from build123d import *

# Parameters (mm, degrees)
SKETCH1_R           = 27.5
SKETCH1_R_2         = 15.5
BOSS_EXTRUDE1_DEPTH = 9
BOSS_EXTRUDE2_DEPTH = 9
SKETCH3_W           = 14
SKETCH3_H           = 2
SKETCH4_W           = 1.6
SKETCH4_H           = 1.9
FILLET1_R           = 10
SKETCH5_W           = 16
SKETCH5_H           = 1
CUT_EXTRUDE1_DEPTH  = 60
SKETCH6_R           = 3
CUT_EXTRUDE2_DEPTH  = 107.495305061
SKETCH7_R           = 3
CUT_EXTRUDE3_DEPTH  = 107.495305061


with BuildPart() as part:
    # Sketch1 → Boss-Extrude1 (new, symmetric)
    with BuildSketch(Plane.XY):
        Circle(SKETCH1_R)
        Circle(SKETCH1_R_2, mode=Mode.SUBTRACT)
    extrude(amount=BOSS_EXTRUDE1_DEPTH, both=True)

    # Sketch2 → Boss-Extrude2 (add, symmetric)
    with BuildSketch(Plane.XY):
        Polygon((-8, 100), (8, 100), (8, 26.310644234), (0, 27.5), (-8, 26.310644234), align=None)
    boss_extrude2 = extrude(amount=BOSS_EXTRUDE2_DEPTH, both=True)

    # Mirror1: Boss-Extrude2 across plane
    add(boss_extrude2.mirror(Plane.ZX))

    # Sketch3 → Cut-Revolve1 (revolve, cut)
    with BuildSketch(Plane(origin=(0, 0, 0), x_dir=(0, 0, -1), z_dir=(1, 0, 0)), mode=Mode.PRIVATE) as cut_revolve1_sk:
        with Locations((-2, 16.5)):
            Rectangle(SKETCH3_W, SKETCH3_H)
    revolve(cut_revolve1_sk.sketch.rotate(Axis((0, 0, 0), (0, 0, -1)), 90), axis=Axis((0, 0, 0), (0, 0, -1)), mode=Mode.SUBTRACT)

    # Sketch4 → Cut-Revolve2 (revolve, cut)
    with BuildSketch(Plane(origin=(0, 0, 0), x_dir=(0, 0, -1), z_dir=(1, 0, 0)), mode=Mode.PRIVATE) as cut_revolve2_sk:
        with Locations((-5.7, 17.95)):
            Rectangle(SKETCH4_W, SKETCH4_H)
    revolve(cut_revolve2_sk.sketch.rotate(Axis((0, 0, 0), (0, 0, -1)), 90), axis=Axis((0, 0, 0), (0, 0, -1)), mode=Mode.SUBTRACT)

    # Fillet1
    fillet1_edges = [part.edges().sort_by_distance(p)[0] for p in [
        (8, 26.310644234, 0),
        (-8, 26.310644234, 0),
        (8, -26.310644234, 0),
        (-8, -26.310644234, 0),
    ]]
    fillet(fillet1_edges, radius=FILLET1_R)

    # Sketch5 → Cut-Extrude1 (cut)
    with BuildSketch(Plane.XZ.offset(100)):
        with Locations((0, 8.5)):
            Rectangle(SKETCH5_W, SKETCH5_H)
        with Locations((0, -8.5)):
            Rectangle(SKETCH5_W, SKETCH5_H)
    cut_extrude1 = extrude(amount=-CUT_EXTRUDE1_DEPTH, mode=Mode.SUBTRACT)

    # Sketch6 → Cut-Extrude2 (cut, through all)
    with BuildSketch(Plane.ZY.offset(8)):
        with Locations(Location((0, 90, 0), (0, 0, 270))):
            Circle(SKETCH6_R)
        with Locations(Location((0, 70, 0), (0, 0, 270))):
            Circle(SKETCH6_R)
    extrude(amount=-CUT_EXTRUDE2_DEPTH, mode=Mode.SUBTRACT)

    # Sketch7 → Cut-Extrude3 (cut, through all)
    with BuildSketch(Plane.ZY.offset(8)):
        with Locations(Location((0, -90, 0), (0, 0, 270))):
            Circle(SKETCH7_R)
        with Locations(Location((0, -70, 0), (0, 0, 270))):
            Circle(SKETCH7_R)
    extrude(amount=-CUT_EXTRUDE3_DEPTH, mode=Mode.SUBTRACT)

    # Mirror2: Cut-Extrude1 across plane
    add(cut_extrude1.mirror(Plane.ZX), mode=Mode.SUBTRACT)


solid = part.part
The listing builds one solid part. Answer for the finished solid, in the listing's coordinates (mm). A direction names the side the tool comes from. Coordinates: 2 decimals unless noted, no trailing zeros. Loops run counter-clockwise (first coordinate to the right, second up) from the corner with the lowest first, then second, coordinate; pieces in that order, holes last.
1) Find the intervals of material crossed by L1, parallel to Y at x = 0, z = 6.25; L2, parallel to Y at x = 1, z = -6.5; L3, parallel to Z at x = 18, y = 5, in increasing order.
2) Find section D-D on y = -71. Write down the section's boundary in (x, z).
3) Find section A-A on z = 0. Give the number of separate pieces and of enclosed holes in the cut face, then the cut area to 3 significant figures.
4) Determine the mould class of faces 6 (the face through (-9.44, 27.73, 0.13)), 7 (the face through (8, -67, -2)), 8 (the face through (-3.794, 17.084, 7.732)) for opening direction Y: pulls with the +Y half, pulls with the -Y half, needs draft (parallel to the pull), parting line crosses it, or undercut.
5) Find section C-C on y = 70. Write down the section's boundary in (x, z), then the cut area to 3 significant figures.
6) A tool of negligible diameter and unlimited length cuts with its end or side. For faces 1 (the face through (-8, 66, 0)), 2 (the face through (0, -70, -8)), 3 (the face through (0, -70, 8)), 4 (the face through (7, 14, -5)), 5 (the face through (-17, 6, 4.9)), from which of +Z, -Z, +X, -X, +Y, -Y can it reach the whole face along a straight path? Write none if from no direction.
7) Flat-ended cylindrical pins translate along their axes: pin 1 Ø9 at (y, z) = (50, -4) entering from -X; pin 2 Ø5 at (y, z) = (70, 0) entering from +X; pin 3 Ø4 at (y, z) = (-13, -5.5) entering from -X; pin 4 Ø9 at (y, z) = (70, -2) entering from +X. Find the tip coordinate at first contact, or state that the pin passes through.
Values:
1. L1: y = -100 to -18.9, 18.9 to 100
1. L2: y = -100 to -15.47, 15.47 to 100
1. L3: z = -9 to 4.9, 6.5 to 9
2. outline: (-8, -8) - (8, -8) - (8, -2.83) - (-8, -2.83) - close; (-8, 2.83) - (8, 2.83) - (8, 8) - (-8, 8) - close
3. separate pieces: 5
3. enclosed holes: 1
3. area: 3,390 mm2
4. face 6: pulls with the +Y half
4. face 7: needs draft
4. face 8: undercut
5. outline: (-8, -8) - (8, -8) - (8, -3) - (-8, -3) - close; (-8, 3) - (8, 3) - (8, 8) - (-8, 8) - close
5. area: 160 mm2
6. face 1: +Z, -Z, -X, +Y
6. face 2: -Z, +X, -X, -Y
6. face 3: +Z, +X, -X, -Y
6. face 4: +Z
6. face 5: none
7. pin 1: stops at x = -8
7. pin 2: passes through
7. pin 3: stops at x = -25.2
7. pin 4: stops at x = 8
